from build123d import *

# Parameters (mm, degrees)
SKETCH_R        = 25
PAD_DEPTH       = 4
SKETCH001_R     = 7
SKETCH001_R_2   = 4
PAD001_DEPTH    = 8
CHAMFER_SIZE    = 2
CHAMFER001_SIZE = 3
CHAMFER002_SIZE = 0.5
SKETCH002_R     = 25
SKETCH002_R_2   = 23
PAD002_DEPTH    = 15


with BuildPart() as part:
    # Sketch → Pad (new body)
    with BuildSketch(Plane.XY):
        Circle(SKETCH_R)
    extrude(amount=PAD_DEPTH)

    # Sketch001 (on Face3 of Pad) → Pad001 (join)
    with BuildSketch(Plane.XY.offset(4)):
        Circle(SKETCH001_R)
        Circle(SKETCH001_R_2, mode=Mode.SUBTRACT)
    extrude(amount=PAD001_DEPTH)

    # Chamfer
    chamfer_edges = [part.edges().sort_by_distance(p)[0] for p in [
        (-25, 0, 0),
    ]]
    chamfer(chamfer_edges, length=CHAMFER_SIZE)

    # Chamfer001
    chamfer001_edges = [part.edges().sort_by_distance(p)[0] for p in [
        (-7, 0, 4),
    ]]
    chamfer(chamfer001_edges, length=CHAMFER001_SIZE)

    # Chamfer002
    chamfer002_edges = [part.edges().sort_by_distance(p)[0] for p in [
        (-4, 0, 12),
    ]]
    chamfer(chamfer002_edges, length=CHAMFER002_SIZE)

    # Sketch002 (on Face7 of Chamfer002) → Pad002 (join)
    with BuildSketch(Plane.XY.offset(4)):
        Circle(SKETCH002_R)
        Circle(SKETCH002_R_2, mode=Mode.SUBTRACT)
    extrude(amount=PAD002_DEPTH)


solid = part.part
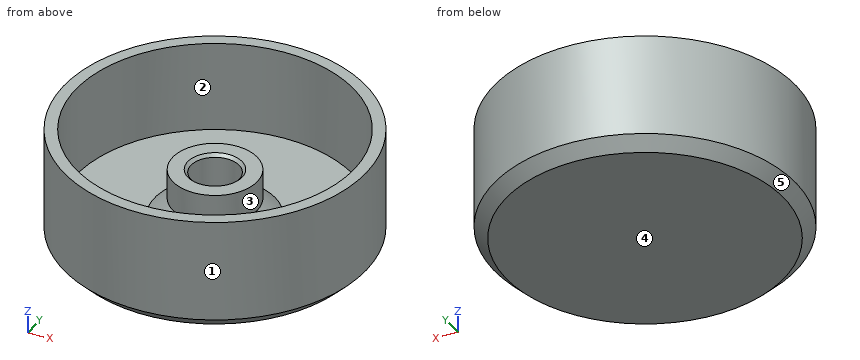
The listing builds one solid part. Answer for the finished solid, in the listing's coordinates (mm). Face numbers are marked on the shaded views. A direction names the side the tool comes from. Give positions to 0.01 mm unless a question says otherwise; leave off trailing zeros. Order: outer loops, then holes, each group sorted by start corner. A loop starts at its lowest first (then second) coordinate and runs counter-clockwise, first axis right, second up. Notation, with made-up numbers: (67.25, 33.5) - (84.25, 33.5) arc R7 cw to (84.25, 40.5) - close; hole circle Ø7 at (-13.75, 22.5). An arc over 180 degrees is marked (long way). One line per item, written item: value. Start each with the question number.
1) Given pin 1 Ø8 at (y, z) = (-16, 7) entering from -X; pin 2 Ø23 at (x, y) = (10, 9) entering from +Z; pin 3 Ø5 at (x, y) = (13.5, -1) entering from +Z; pin 4 Ø1.5 at (y, z) = (-8.5, 5) entering from -X, each flat-ended and moving along its own axis, determine where each tip first touches the part or whether it passes through.
2) Find the intervals of material crossed by L1, parallel to Y at x = 0, z = 8.5; L2, parallel to Y at x = -5, z = 10; L3, parallel to Y at x = 0, z = 6.5, in increasing order.
3) The mould has two halves that part along X. Classify the marked faces 3, 4 and 5: released by +X, released by -X, zero draft, split by the parting line, or undercut.
4) A tool of negligible diameter and unlimited length cuts with its end or side. For the marked faces 1 and 2, from which of +Z, -Z, +X, -X, +Y, -Y can it reach the whole face along a straight path? Write none if from no direction.
5) A cutting plane is placed at A-A on y = 0. Give the vertices of the cut face in (x, z).
6) A cutting plane is placed at C-C on z = 14. Give the vertices of the cut face in (x, y).
Answer sheet:
1. pin 1: stops at x = -21.93
1. pin 2: stops at z = 19
1. pin 3: stops at z = 4
1. pin 4: stops at x = -23.77
2. L1: y = -25 to -23, -7 to -4, 4 to 7, 23 to 25
2. L2: y = -24.49 to -22.45, -4.9 to 4.9, 22.45 to 24.49
2. L3: y = -25 to -23, -7.5 to -4, 4 to 7.5, 23 to 25
3. face 3: undercut
3. face 4: zero draft
3. face 5: split by the parting line
4. face 1: +Z, -Z
4. face 2: +Z
5. outline: (-25, 2) - (-23, 0) - (23, 0) - (25, 2) - (25, 19) - (23, 19) - (23, 4) - (10, 4) - (7, 7) - (7, 12) - (4.5, 12) - (4, 11.5) - (4, 4) - (-4, 4) - (-4, 11.5) - (-4.5, 12) - (-7, 12) - (-7, 7) - (-10, 4) - (-23, 4) - (-23, 19) - (-25, 19) - close
6. outline: circle Ø50 at (0, 0); hole circle Ø46 at (0, 0)
